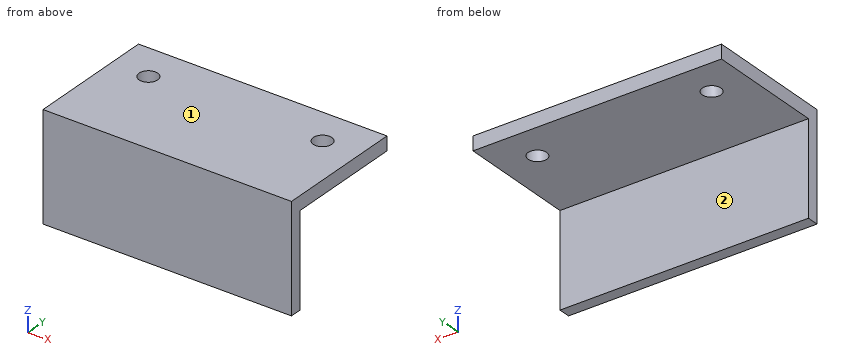
from build123d import *

# Parameters (mm, degrees)
SKETCH002_W     = 53.5
SKETCH002_H     = 28
PAD_DEPTH       = 3
SKETCH_R        = 2
POCKET_DEPTH    = 5
SKETCH001_R     = 2
POCKET001_DEPTH = 5
SKETCH003_W     = 53.5
SKETCH003_H     = 2.5
PAD001_DEPTH    = 20


with BuildPart() as part:
    # Sketch002 → Pad (new body)
    with BuildSketch(Plane.XY):
        with Locations((18.75, -6)):
            Rectangle(SKETCH002_W, SKETCH002_H)
    extrude(amount=PAD_DEPTH)

    # Sketch → Pocket (cut)
    with BuildSketch(Plane.XY):
        Circle(SKETCH_R)
    extrude(amount=POCKET_DEPTH, mode=Mode.SUBTRACT)

    # Sketch001 → Pocket001 (cut)
    with BuildSketch(Plane.XY):
        with Locations((37.5, 0)):
            Circle(SKETCH001_R)
    extrude(amount=POCKET001_DEPTH, mode=Mode.SUBTRACT)

    # Sketch003 → Pad001 (join)
    with BuildSketch(Plane.XY):
        with Locations((18.75, -18.75)):
            Rectangle(SKETCH003_W, SKETCH003_H)
    extrude(amount=-PAD001_DEPTH)


solid = part.part
Verification items for the finished model (mm, model axes). Face numbers are marked on the shaded views. A direction names the side the tool comes from. Coordinates: 2 decimals unless noted, no trailing zeros. Loops run counter-clockwise (first coordinate to the right, second up) from the corner with the lowest first, then second, coordinate; pieces in that order, holes last. Notation, with made-up numbers: (48.5, -20) -> (105.5, -20) arc R24 ccw to (105.5, 3) -> close; hole circle Ø3 at (66.25, 60.5). An arc over 180 degrees is marked (long way). Answer as a JSON object with one key per item and string values. Group by question number.
Item 1: Depth check by flat-ended pin: pin 1 (8 mm diameter, centred on x = 27, z = -5, fed in from +Y); pin 2 (4 mm diameter, centred on x = 12.5, y = -0.5, fed in from -Z); pin 3 (6.5 mm diameter, centred on x = 37.5, y = 0, fed in from +Z). Enter the tip coordinate at first touch or a pass-through.
Item 2: Tool access check on the marked faces 1 and 2. Record the directions out of +Z, -Z, +X, -X, +Y, -Y that give a thin tool (end or side, any length) a straight path to the whole face; none if there is none.
Item 3: Sectioned sample at D-D on z = -9.25. Record the boundary of the cut face in (x, y).
Item 4: Sectioned sample at A-A on x = 37.5. Record the boundary of the cut face in (y, z), plus the area to 3 significant figures.
Item 5: Sectioned sample at C-C on z = 1. Record the boundary of the cut face in (x, y).
Item 6: Scan lines: probe 1 along X at (y, z) = (0, 0.6); probe 2 along Z at (x, y) = (37, -9.5); probe 3 along Y at (x, z) = (18, -3). Record each from-to range of solid material in increasing order.
Item 7: Sectioned sample at B-B on y = 0. Record the boundary of the cut face in (x, z), plus the area to 4 significant figures.
Evaluation:
{
 "1": {"pin 1": "stops at y = -17.5", "pin 2": "stops at z = 0", "pin 3": "stops at z = 3"},
 "2": {"face 1": "+Z, +X, -X, +Y, -Y", "face 2": "-Z, +X, -X, +Y"},
 "3": {"outline": "(-8, -20) -> (45.5, -20) -> (45.5, -17.5) -> (-8, -17.5) -> close"},
 "4": {"outline": "(-20, -20) -> (-17.5, -20) -> (-17.5, 0) -> (-2, 0) -> (-2, 3) -> (-20, 3) -> close; (2, 0) -> (8, 0) -> (8, 3) -> (2, 3) -> close", "area": "122 mm²"},
 "5": {"outline": "(-8, -20) -> (45.5, -20) -> (45.5, 8) -> (-8, 8) -> close; hole circle Ø4 at (0, 0); hole circle Ø4 at (37.5, 0)"},
 "6": {"probe 1": "x = -8 to -2, 2 to 35.5, 39.5 to 45.5", "probe 2": "z = 0 to 3", "probe 3": "y = -20 to -17.5"},
 "7": {"outline": "(-8, 0) -> (-2, 0) -> (-2, 3) -> (-8, 3) -> close; (2, 0) -> (35.5, 0) -> (35.5, 3) -> (2, 3) -> close; (39.5, 0) -> (45.5, 0) -> (45.5, 3) -> (39.5, 3) -> close", "area": "136.5 mm²"}
}
